from build123d import *

# Parameters (mm, degrees)
SKETCH1_W           = 28
SKETCH1_H           = 28
BOSS_EXTRUDE1_DEPTH = 2
SKETCH2_R           = 14
BOSS_EXTRUDE2_DEPTH = 53
SKETCH3_R           = 6
CUT_EXTRUDE1_DEPTH  = 56


with BuildPart() as part:
    # Sketch1 → Boss-Extrude1 (new body)
    with BuildSketch(Plane.XY):
        Rectangle(SKETCH1_W, SKETCH1_H)
    extrude(amount=BOSS_EXTRUDE1_DEPTH)

    # Sketch2 → Boss-Extrude2 (add)
    with BuildSketch(Plane.XY.offset(2)):
        Circle(SKETCH2_R)
    extrude(amount=BOSS_EXTRUDE2_DEPTH)

    # Sketch3 → Cut-Extrude1 (cut, through all)
    with BuildSketch(Plane(origin=(0, 0, 0), x_dir=(-1, 0, 0), z_dir=(0, 0, -1))):
        Circle(SKETCH3_R)
    extrude(amount=-CUT_EXTRUDE1_DEPTH, mode=Mode.SUBTRACT)


solid = part.part
Read the model definition and answer for the solid it produces. Units are mm, in the model's axes. A direction names the side the tool comes from. Give positions to 0.01 mm unless a question says otherwise; leave off trailing zeros. Write each loop counter-clockwise with the first axis right and the second up, starting at its lowest first coordinate (ties: lowest second). Pieces come first, ordered by that corner, then holes. Notation, with made-up numbers: M 10,41.5 L 24,41.5 A9 ccw 24,47.5 Z; hole C 38.25,58.5 d11. An arc over 180 degrees is marked long. One line per item, written item: value. Start each with the question number.
(1) Find section C-C (y = 7). Determine the outline of the cut face in (x, z).
(2) Find the intervals of material crossed by line 1 (Y direction, x = 0, z = 17.5); line 2 (X direction, y = 0.25, z = 27.5); line 3 (Y direction, x = 3.25, z = 9), in increasing order.
(3) Find section D-D (z = 30). Determine the outline of the cut face in (x, y), plus the area to 3 significant figures.
(4) Find section A-A (y = -2). Determine the outline of the cut face in (x, z), plus the area to 3 significant figures.
(5) Flat-ended cylindrical pins translate along their axes: pin 1 Ø1 at (x, z) = (-5, 38.5) entering from -Y; pin 2 Ø3 at (y, z) = (-4, 14) entering from -X (3 decimals); pin 3 Ø1.5 at (y, z) = (4, 29.5) entering from +X. Find the tip coordinate at first contact, or state that the pin passes through.
(6) Determine the mould class of faces 1 (the cylindrical face through (6, 0, 27)), 2 (the flat face through (-14, 0, 1)), 3 (the cylindrical face through (12.932, -5.362, 28.129)), 4 (the flat face through (-11, -11, 2)) for opening direction X: pulls with the +X half, pulls with the -X half, needs draft (parallel to the pull), parting line crosses it, or undercut.
(7) A tool of negligible diameter and unlimited length cuts with its end or side. For faces 5 (the flat face through (11, -11, 2)), 6 (the flat face through (-11, 11, 2)), 7 (the flat face through (0, 14, 1)), 8 (the flat face through (11, 11, 2)), from which of +Z, -Z, +X, -X, +Y, -Y can it reach the whole face along a straight path? Write none if from no direction.
Results below:
1. outline: M -14,0 L 14,0 L 14,2 L 12.12,2 L 12.12,55 L -12.12,55 L -12.12,2 L -14,2 Z
2. line 1: y = -14 to -6, 6 to 14
2. line 2: x = -14 to -5.99, 5.99 to 14
2. line 3: y = -13.62 to -5.04, 5.04 to 13.62
3. outline: C 0,0 d28; hole C 0,0 d12
3. area: 503 mm^2
4. outline: M -14,0 L -5.66,0 L -5.66,55 L -13.86,55 L -13.86,2 L -14,2 Z; M 5.66,0 L 14,0 L 14,2 L 13.86,2 L 13.86,55 L 5.66,55 Z
4. area: 903 mm^2
5. pin 1: stops at y = -13.26
5. pin 2: stops at x = -13.775
5. pin 3: stops at x = 13.62
6. face 1: undercut
6. face 2: pulls with the -X half
6. face 3: parting line crosses it
6. face 4: needs draft
7. face 5: +Z, +X, -Y
7. face 6: +Z, -X, +Y
7. face 7: +Z, -Z, +X, -X, +Y
7. face 8: +Z, +X, +Y
